The figure shows three views and two pictorial views of one solid part (mm, origin at its lowest corner). Answer the questions. A direction names the side the tool comes from. Coordinates: 2 decimals unless noted, no trailing zeros. Loops run counter-clockwise (first coordinate to the right, second up) from the corner with the lowest first, then second, coordinate; pieces in that order, holes last. Notation, with made-up numbers: M 2,73 L 45,73 A21 cw 45,79 Z; hole C -38,65.25 d1. An arc over 180 degrees is marked long. One line per item, written item: value. Start each with the question number.
1. Consider probe 1 along X at (y, z) = (28.75, 5.5); probe 2 along X at (y, z) = (12.25, 36); probe 3 along Z at (x, y) = (4.25, 11.75). Determine where each line is inside the solid, lowest interval first.
2. For the marked faces 5, 6 and 7, determine the directions among +Z, -Z, +X, -X, +Y, -Y from which every point of the face is accessible in a straight line to the end or side of a thin tool.
3. The part is cut by section C-C (x = 12.25). Write down the section's boundary in (y, z).
4. A flat-ended cylindrical pin translates along its axis: pin 1 (1.8 mm diameter, centred on x = 2.5, y = 13, fed in from -Z). Find the tip coordinate at first contact, or state that the pin passes through.
5. The part is cut by section B-B (y = 18). Write down the section's boundary in (x, z), then the cut area to 3 significant figures.
6. The part is cut by section A-A (z = 48). Write down the section's boundary in (x, y).
7. Determine the mould class of the marked faces 1, 2, 3 and 4 for opening direction X: +X half, -X half, draft (parallel to the pull), parting line (faces both ways), or undercut.
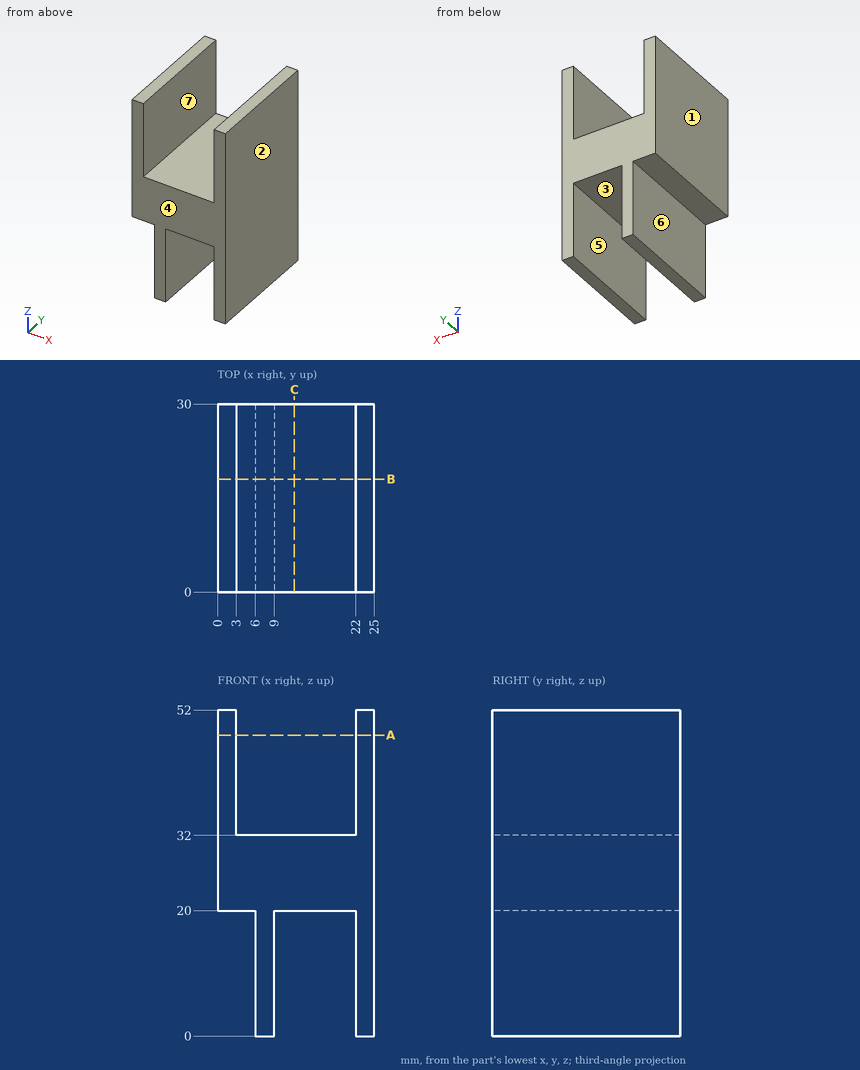
Answer block:
1. probe 1: x = 6 to 9, 22 to 25
1. probe 2: x = 0 to 3, 22 to 25
1. probe 3: z = 20 to 32
2. face 5: -Z, +Y, -Y
2. face 6: -Z, -X, +Y, -Y
2. face 7: +Z, +Y, -Y
3. outline: M 0,20 L 30,20 L 30,32 L 0,32 Z
4. pin 1: stops at z = 20
5. outline: M 0,20 L 6,20 L 6,0 L 9,0 L 9,20 L 22,20 L 22,0 L 25,0 L 25,52 L 22,52 L 22,32 L 3,32 L 3,52 L 0,52 Z
5. area: 540 mm2
6. outline: M 0,0 L 3,0 L 3,30 L 0,30 Z; M 22,0 L 25,0 L 25,30 L 22,30 Z
7. face 1: -X half
7. face 2: +X half
7. face 3: undercut
7. face 4: draft
